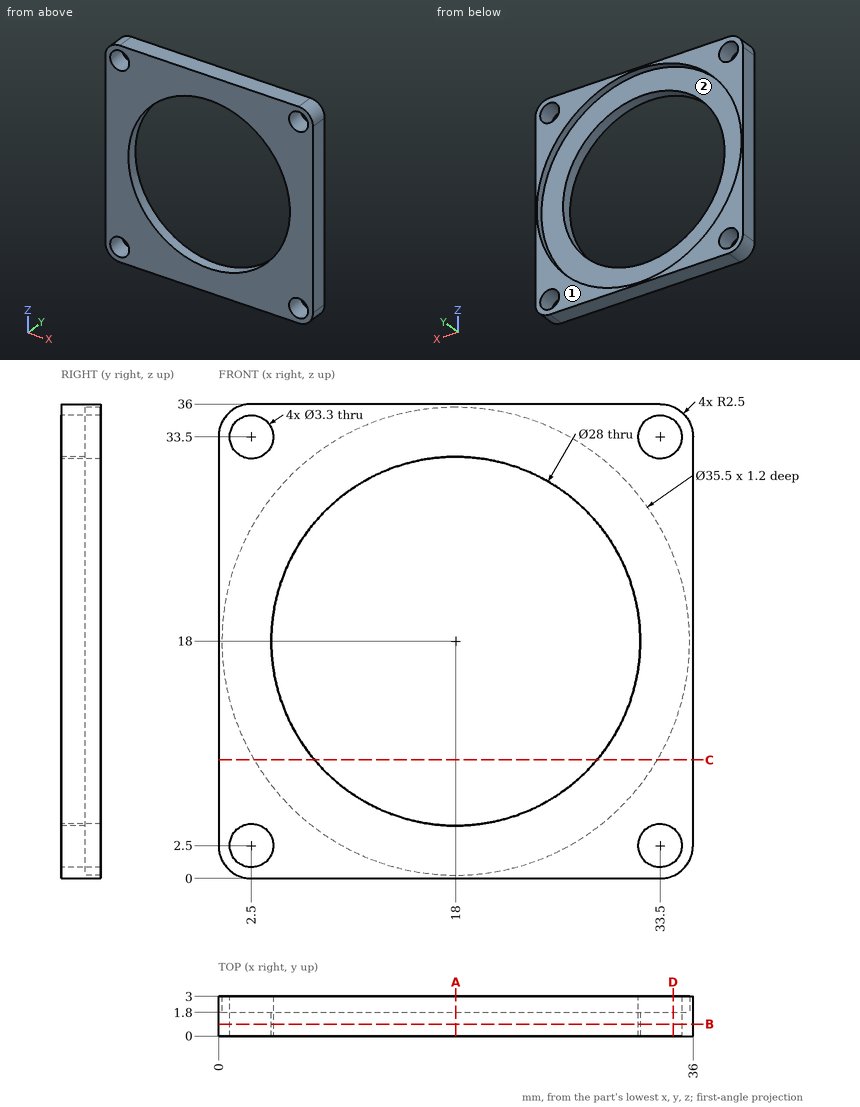
Job drawing, mm, ordinate dimensions from the low corner. One solid piece. Coordinates: 2 decimals unless noted, no trailing zeros. Write each loop counter-clockwise with the first axis right and the second up, starting at its lowest first coordinate (ties: lowest second). Pieces come first, ordered by that corner, then holes. Notation, with made-up numbers: (77, -13) -> (91, -13) arc R28 cw to (91, 14) -> close; hole circle Ø3 at (5.5, -39.75). An arc over 180 degrees is marked (long way). Use CSV: the item, a comma, the result in double quotes. Start each with the question number.
Item 1: Band-saw the part on D-D, the plane x = 34.5. Write the cut outline in (y, z), plus the area to 3 significant figures.
Item 2: Drop a flat-ended pin along its axis: P1, Ø5, axis at x = 26.5, z = 4, coming from the -Y side. Give the stop position or say it passes through.
Item 3: Band-saw the part on B-B, the plane y = 0.9. Write the cut outline in (x, z), plus the area to 3 significant figures.
Item 4: Two-plate mould, pull along X, no slides. Class the marked faces 1 and 2: +X half, -X half, draft (parallel to the pull), parting line (faces both ways), or undercut.
Item 5: Band-saw the part on A-A, the plane x = 18. Write the cut outline in (y, z).
Item 6: Band-saw the part on C-C, the plane z = 9. Write the cut outline in (x, y), plus the area to 3 significant figures.
Item 7: Wall check: probe 1 along Z at (x, y) = (18, 2.6); probe 2 along X at (y, z) = (2.6, 32); probe 3 along X at (y, z) = (1.2, 18). Give the ranges that are in metal, low to high.
Response values:
1,outline,"(0, 0.21) -> (3, 0.21) -> (3, 1.19) -> (0, 1.19) -> close; (0, 3.81) -> (3, 3.81) -> (3, 11.46) -> (1.8, 11.46) -> (1.8, 24.54) -> (3, 24.54) -> (3, 32.19) -> (0, 32.19) -> close; (0, 34.81) -> (3, 34.81) -> (3, 35.79) -> (0, 35.79) -> close"
1,area,"75.3 mm2"
2,P1,"stops at y = 0"
3,outline,"(0, 2.5) arc R2.5 ccw to (2.5, 0) -> (33.5, 0) arc R2.5 ccw to (36, 2.5) -> (36, 33.5) arc R2.5 ccw to (33.5, 36) -> (2.5, 36) arc R2.5 ccw to (0, 33.5) -> close; hole circle Ø3.3 at (2.5, 2.5); hole circle Ø3.3 at (2.5, 33.5); hole circle Ø28 at (18, 18); hole circle Ø3.3 at (33.5, 2.5); hole circle Ø3.3 at (33.5, 33.5)"
3,area,"641 mm2"
4,face 1,"draft"
4,face 2,"undercut"
5,outline,"(0, 0) -> (3, 0) -> (3, 0.25) -> (1.8, 0.25) -> (1.8, 4) -> (0, 4) -> close; (0, 32) -> (1.8, 32) -> (1.8, 35.75) -> (3, 35.75) -> (3, 36) -> (0, 36) -> close"
6,outline,"(0, 0) -> (7.28, 0) -> (7.28, 1.8) -> (2.7, 1.8) -> (2.7, 3) -> (0, 3) -> close; (28.72, 0) -> (36, 0) -> (36, 3) -> (33.3, 3) -> (33.3, 1.8) -> (28.72, 1.8) -> close"
6,area,"32.7 mm2"
7,probe 1,"z = 0 to 0.25, 35.75 to 36"
7,probe 2,"x = 0 to 1.81, 3.19 to 7.09, 28.91 to 32.81, 34.19 to 36"
7,probe 3,"x = 0 to 4, 32 to 36"
